Work out the finished part from the listing and answer in its coordinate system (mm). Face numbers are marked on the shaded views. Give positions to 0.01 mm unless a question says otherwise; leave off trailing zeros. Order: outer loops, then holes, each group sorted by start corner. A loop starts at its lowest first (then second) coordinate and runs counter-clockwise, first axis right, second up.
Autodesk Inventor part; units mm, degrees
ref_plane "YZ Plane" through (0, 0, 0) normal (1, 0, 0) x (0, 1, 0)
ref_plane "XZ Plane" through (0, 0, 0) normal (0, 1, 0) x (-1, 0, 0)
ref_plane "XY Plane" through (0, 0, 0) normal (0, 0, 1) x (1, 0, 0)
sketch "Sketch1" plane through (0, 0, 0) normal (0, 1, 0) x (-1, 0, 0)
  circle A0 centre (0, 0) radius 7.95
  dimension "d0" = 15.9
extrude "Extrusion1" add sketch "Sketch1" along normal blind 60.4
sketch "Sketch2" plane through (0, 0, 0) normal (0, -1, 0) x (1, 0, 0)
  circle A0 centre (0, 0) radius 2.65
  dimension "d3" = 5.3
extrude "Extrusion2" add sketch "Sketch2" along normal blind 2
sketch "Sketch3" plane through (0, -2, 0) normal (0, -1, 0) x (1, 0, 0)
  circle A0 centre (0, 0) radius 0.6
  dimension "d6" = 1.2
extrude "Extrusion3" add sketch "Sketch3" along normal blind 21
sketch "Sketch4" plane through (0, 60.4, 0) normal (0, 1, 0) x (1, 0, 0)
  circle A0 centre (0, 0) radius 7.45
  dimension "d9" = 14.9
extrude "Extrusion4" cut sketch "Sketch4" against normal blind 60
properties part number "Syringe_moreaccurate_ENES100_OSV-spencermical-4-52pm-3-5-16-saturday"
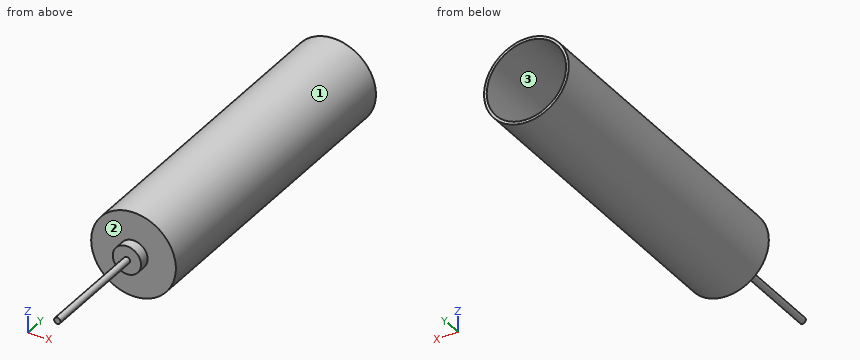
1. The part is cut by section C-C (y = -15.5). Write down the section's boundary in (x, z).
Findings below:
outline: circle Ø1.2 at (0, 0)
2. The mould has two halves that part along Z. Classify the marked faces 1, 2 and 3: pulls with the +Z half, pulls with the -Z half, needs draft (parallel to the pull), parting line crosses it, or undercut.
Findings below:
face 1: parting line crosses it
face 2: needs draft
face 3: undercut
3. Straight lines are drawn through the part: probe 1 along Z at (x, y) = (0, 15.5); probe 2 along Y at (x, z) = (-5, 2). For each, find the intervals that lie inside material, in ascending order.
Findings below:
probe 1: z = -7.95 to -7.45, 7.45 to 7.95
probe 2: y = 0 to 0.4
4. The part is cut by section A-A (y = 39). Write down the section's boundary in (x, z), then the cut area to 3 significant figures.
Findings below:
outline: circle Ø15.9 at (0, 0); hole circle Ø14.9 at (0, 0)
area: 24.2 mm2
5. Given P1, Ø3, axis at y = 11.5, z = -6.5, coming from the -X side; P2, Ø8, axis at y = 37.5, z = -5.5, coming from the +X side; P3, Ø1, axis at x = -1.5, y = 7, coming from the -Z side, each flat-ended and moving along its own axis, determine where each tip first touches the part or whether it passes through.
Findings below:
P1: stops at x = -6.18
P2: stops at x = 7.81
P3: stops at z = -7.89
6. The part is cut by section B-B (x = 3.75). Write down the section's boundary in (y, z), then the cut area to 3 significant figures.
Findings below:
outline: (0, -7.01) - (60.4, -7.01) - (60.4, -6.44) - (0.4, -6.44) - (0.4, 6.44) - (60.4, 6.44) - (60.4, 7.01) - (0, 7.01) - close
area: 74.3 mm2
